Geometry: final body of the model. Coordinates: model frame, mm. Face numbers are marked on the shaded views. A direction names the side the tool comes from. Round coordinates to 2 decimals unless told otherwise and drop trailing zeros. Loops run counter-clockwise (first coordinate to the right, second up) from the corner with the lowest first, then second, coordinate; pieces in that order, holes last. Notation, with made-up numbers: (30.25, 88) - (78.25, 88) arc R28 cw to (78.25, 107) - close; hole circle Ø11 at (81.25, 73.5). An arc over 180 degrees is marked (long way). Use CSV: the item, a comma, the result in double quotes.
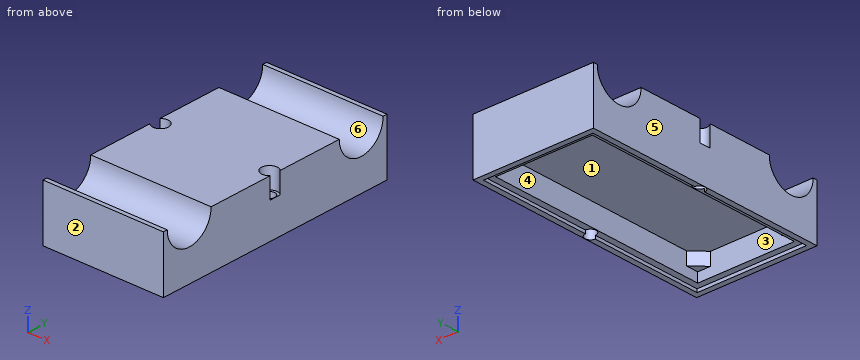
from build123d import *

# Parameters (mm, degrees)
SKETCH1_W           = 38
SKETCH1_H           = 78
BOSS_EXTRUDE1_DEPTH = 10
SKETCH2_W           = 30.5
SKETCH2_H           = 70.5
CUT_EXTRUDE1_DEPTH  = 8
BOSS_EXTRUDE2_DEPTH = 4
SKETCH4_W           = 38
SKETCH4_H           = 78
BOSS_EXTRUDE3_DEPTH = 7.5
SKETCH5_R           = 7.65
CUT_EXTRUDE2_DEPTH  = 89.511298714
SKETCH6_W           = 34.5
SKETCH6_H           = 74.5
SKETCH6_W_2         = 30.5
SKETCH6_H_2         = 70.5
CUT_EXTRUDE3_DEPTH  = 1
SKETCH7_R           = 1.725
CUT_EXTRUDE5_DEPTH  = 89.511298714
SKETCH8_R           = 2.5
CUT_EXTRUDE6_DEPTH  = 6.5


with BuildPart() as part:
    # Sketch1 → Boss-Extrude1 (new body)
    with BuildSketch(Plane.XY):
        with Locations((19, 39)):
            Rectangle(SKETCH1_W, SKETCH1_H)
    extrude(amount=BOSS_EXTRUDE1_DEPTH)

    # Sketch2 → Cut-Extrude1 (cut)
    with BuildSketch(Plane(origin=(0, 0, 0), x_dir=(-1, 0, 0), z_dir=(0, 0, -1))):
        with Locations((-19, 39)):
            Rectangle(SKETCH2_W, SKETCH2_H)
    extrude(amount=-CUT_EXTRUDE1_DEPTH, mode=Mode.SUBTRACT)

    # Sketch3 → Boss-Extrude2 (add)
    with BuildSketch(Plane(origin=(0, 0, 8), x_dir=(-1, 0, 0), z_dir=(0, 0, -1))):
        Polygon((-30.25, 74.25), (-34.25, 70.25), (-34.25, 74.25), align=None)
        Polygon((-3.75, 70.25), (-3.75, 74.25), (-7.75, 74.25), align=None)
        Polygon((-3.75, 7.75), (-3.75, 3.75), (-7.75, 3.75), align=None)
        Polygon((-34.25, 7.75), (-34.25, 3.75), (-30.25, 3.75), align=None)
    extrude(amount=BOSS_EXTRUDE2_DEPTH)

    # Sketch4 → Boss-Extrude3 (add)
    with BuildSketch(Plane.XY.offset(10)):
        with Locations((19, 39)):
            Rectangle(SKETCH4_W, SKETCH4_H)
    extrude(amount=BOSS_EXTRUDE3_DEPTH)

    # Sketch5 → Cut-Extrude2 (cut, through all)
    with BuildSketch(Plane(origin=(38, 0, 0), x_dir=(0, 0, -1), z_dir=(1, 0, 0))):
        with Locations((-17.5, 9)):
            Circle(SKETCH5_R)
        with Locations((-17.5, 69)):
            Circle(SKETCH5_R)
    extrude(amount=-CUT_EXTRUDE2_DEPTH, mode=Mode.SUBTRACT)

    # Sketch6 → Cut-Extrude3 (cut)
    with BuildSketch(Plane(origin=(0, 0, 0), x_dir=(-1, 0, 0), z_dir=(0, 0, -1))):
        with Locations((-19, 39)):
            Rectangle(SKETCH6_W, SKETCH6_H)
        with Locations((-19, 39)):
            Rectangle(SKETCH6_W_2, SKETCH6_H_2, mode=Mode.SUBTRACT)
    extrude(amount=-CUT_EXTRUDE3_DEPTH, mode=Mode.SUBTRACT)

    # Sketch7 → Cut-Extrude5 (cut, through all)
    with BuildSketch(Plane.XY.offset(17.5)):
        with Locations((1.8, 39)):
            Circle(SKETCH7_R)
        with Locations((36.2, 39)):
            Circle(SKETCH7_R)
    extrude(amount=-CUT_EXTRUDE5_DEPTH, mode=Mode.SUBTRACT)

    # Sketch8 → Cut-Extrude6 (cut)
    with BuildSketch(Plane.XY.offset(17.5)):
        with Locations((1.8, 39)):
            Circle(SKETCH8_R)
        with Locations((36.2, 39)):
            Circle(SKETCH8_R)
    extrude(amount=-CUT_EXTRUDE6_DEPTH, mode=Mode.SUBTRACT)


solid = part.part
Item 1: Section A-A on y = 39. Return the cut outline in (x, z) (3 decimals), plus the area to 3 significant figures.
Final values:
outline,"(0, 0) - (0.075, 0) - (0.075, 11) - (0, 11) - close; (3.525, 1) - (3.75, 1) - (3.75, 8) - (34.25, 8) - (34.25, 1) - (34.475, 1) - (34.475, 11) - (33.7, 11) - (33.7, 17.5) - (4.3, 17.5) - (4.3, 11) - (3.525, 11) - close; (37.925, 0) - (38, 0) - (38, 11) - (37.925, 11) - close"
area,"289 mm²"
Item 2: Mould query, pull axis X, two halves, no side actions, for the marked faces 3, 4, 5 and 6. Classes: released by +X, released by -X, zero draft, split by the parting line, or undercut.
Final values:
face 3,"undercut"
face 4,"undercut"
face 5,"released by -X"
face 6,"zero draft"
Item 3: Section C-C on z = 13.25. Return the cut outline in (x, y), plus the area to 3 significant figures.
Final values:
outline,"(0, 0) - (38, 0) - (38, 2.64) - (0, 2.64) - close; (0, 15.36) - (38, 15.36) - (38, 37.27) arc R2.5 cw (long way) to (38, 40.73) - (38, 62.64) - (0, 62.64) - (0, 40.73) arc R2.5 cw (long way) to (0, 37.27) - close; (0, 75.36) - (38, 75.36) - (38, 78) - (0, 78) - close"
area,"1,960 mm²"
Item 4: Pin query (flat end, axial travel): P1, Ø2, axis at x = 5.5, y = 6, coming from the -Z side; P2, Ø3, axis at x = 12, y = 65, coming from the +Z side; P3, Ø10, axis at x = 27, y = 31, coming from the -Z side. Return the tip coordinate at first contact, or that it passes through.
Final values:
P1,"stops at z = 4"
P2,"stops at z = 12.18"
P3,"stops at z = 8"
Item 5: Section B-B on x = 6. Return the cut outline in (y, z).
Final values:
outline,"(0, 0) - (1.75, 0) - (1.75, 1) - (3.75, 1) - (3.75, 4) - (5.5, 4) - (5.5, 8) - (72.5, 8) - (72.5, 4) - (74.25, 4) - (74.25, 1) - (76.25, 1) - (76.25, 0) - (78, 0) - (78, 17.5) - (76.65, 17.5) arc R7.65 cw to (61.35, 17.5) - (16.65, 17.5) arc R7.65 cw to (1.35, 17.5) - (0, 17.5) - close"
Item 6: Section D-D on y = 21.5. Return the cut outline in (x, z).
Final values:
outline,"(0, 0) - (1.75, 0) - (1.75, 1) - (3.75, 1) - (3.75, 8) - (34.25, 8) - (34.25, 1) - (36.25, 1) - (36.25, 0) - (38, 0) - (38, 17.5) - (0, 17.5) - close"
Item 7: Material intervals for line 1 (Y direction, x = 30.5, z = 16.75); line 2 (X direction, y = 72.5, z = 1.5); line 3 (Y direction, x = 36.2, z = 13.5), sorted ascending.
Final values:
line 1,"y = 0 to 1.39, 16.61 to 61.39, 76.61 to 78"
line 2,"x = 0 to 3.75, 34.25 to 38"
line 3,"y = 0 to 2.48, 15.52 to 36.5, 41.5 to 62.48, 75.52 to 78"
Item 8: Reachability of the marked faces 1 and 2 from +Z, -Z, +X, -X, +Y, -Y: full face, straight path, thin tool, end or side. Return the list, or none.
Final values:
face 1,"-Z"
face 2,"+Z, -Z, +X, -X, -Y"
